For this review, take the finished solid that the model builds, in its own axes (mm). Face numbers are marked on the shaded views. A direction names the side the tool comes from. Give positions to 0.01 mm unless a question says otherwise; leave off trailing zeros. Loops run counter-clockwise (first coordinate to the right, second up) from the corner with the lowest first, then second, coordinate; pieces in that order, holes last. Notation, with made-up numbers: (80, -37.75) -> (108, -37.75) arc R15 ccw to (108, -19.75) -> close; hole circle Ø10 at (72, 19.25). An arc over 180 degrees is marked (long way). Answer as CSV lines item,"result". Start each with the question number.
Item 1: Add section D-D on y = 12.5. State the section outline as (x, z) points, plus the area to 3 significant figures.
Item 2: Machinability: for the marked faces 4, 5 and 6, which of the approach directions +Z, -Z, +X, -X, +Y, -Y give a long, thin tool a straight path to every point of the face, cutting with its end or side? Answer none if there is none.
Item 3: Clearance check with flat-ended pins moving along their axes: P1, Ø2, axis at x = 16.5, z = 13, coming from the +Y side; P2, Ø5.5, axis at x = -4, z = 16, coming from the -Y side; P3, Ø6.5, axis at y = 18.5, z = 13.5, coming from the +X side. State where each tip first meets the part, or that it passes through.
Item 4: Add section A-A on x = 0. State the section outline as (y, z) points.
Item 5: Add section B-B on y = 0. State the section outline as (x, z) points.
Item 6: Add section C-C on z = 17. State the section outline as (x, y) points.
Item 7: The part is to be moulded in two halves that separate along Y. For the marked faces 1, 2 and 3, say which applies: +Y half, -Y half, draft (parallel to the pull), parting line (faces both ways), or undercut.
Item 8: For L1, parallel to X at y = 0, z = 16.3; L2, parallel to Y at x = 16, z = 13.75; L3, parallel to Y at x = -21, z = 15, list the stretches that pass through material, from the lowest coordinate up. Write a range as from..to.
```python
from build123d import *

# Parameters (mm, degrees)
SKETCH005_R             = 30
PAD002_DEPTH            = 13
SKETCH006_R             = 29
POCKET001_DEPTH         = 3.5
SKETCH007_R             = 27.5
PAD003_DEPTH            = 3.5
SKETCH010_W             = 44
SKETCH010_H             = 22
POCKET003_DEPTH         = 7
SKETCH018_W             = 32
SKETCH018_H             = 40
POCKET011_DEPTH         = 13
SKETCH020_W             = 5
SKETCH020_H             = 3
POCKET012_DEPTH         = 8
SKETCH023_R             = 2.25
POCKET015_DEPTH         = 20
BODY002_PLACEMENT_ANGLE = 90


with BuildPart() as part:
    # Sketch005 → Pad002 (new body)
    with BuildSketch(Plane.XY):
        Circle(SKETCH005_R)
    extrude(amount=PAD002_DEPTH)

    # Sketch006 (on Face3 of Pad002) → Pocket001 (cut)
    with BuildSketch(Plane.XY.offset(13)):
        Circle(SKETCH006_R)
    extrude(amount=-POCKET001_DEPTH, mode=Mode.SUBTRACT)

    # Sketch007 (on Face5 of Pocket001) → Pad003 (join)
    with BuildSketch(Plane.XY.offset(9.5)):
        Circle(SKETCH007_R)
    extrude(amount=PAD003_DEPTH)

    # Sketch010 (on Face7 of Pad003) → Pocket003 (cut)
    with BuildSketch(Plane.XY.offset(13)):
        Rectangle(SKETCH010_W, SKETCH010_H)
    extrude(amount=-POCKET003_DEPTH, mode=Mode.SUBTRACT)

    # Sketch018 (on Face7 of Pocket003) → Pocket011 (cut)
    with BuildSketch(Plane.XY.offset(13)):
        Rectangle(SKETCH018_W, SKETCH018_H)
    extrude(amount=-POCKET011_DEPTH, mode=Mode.SUBTRACT)

    # Sketch020 (on Face5 of Pocket011) → Pocket012 (cut)
    with BuildSketch(Plane(origin=(0, -20, 0), x_dir=(-1, 0, 0), z_dir=(0, 1, 0))):
        with Locations((0, 11.5)):
            Rectangle(SKETCH020_W, SKETCH020_H)
    extrude(amount=-POCKET012_DEPTH, mode=Mode.SUBTRACT)

    # Sketch023 (on Face9 of Pocket012) → Pocket015 (cut)
    with BuildSketch(Plane.XY.offset(13)):
        with Locations((-19.108778, -14.520833)):
            Circle(SKETCH023_R)
        with Locations((0, 24)):
            Circle(SKETCH023_R)
        with Locations((19.108778, -14.520833)):
            Circle(SKETCH023_R)
    extrude(amount=-POCKET015_DEPTH, mode=Mode.SUBTRACT)


with BuildPart() as part_1:
    # Body002 placement: moved
    add(part.part.moved(Location((0, 0, 5))).rotate(Axis((0, 0, 5), (0, 0, 1)), BODY002_PLACEMENT_ANGLE))


solid = part_1.part
```
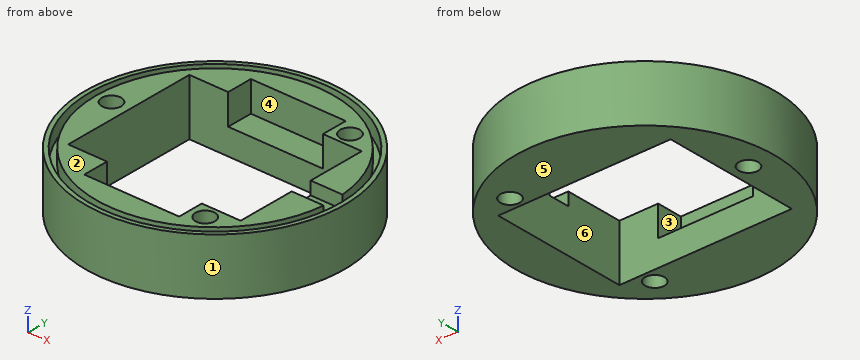
Computed values:
1,outline,"(-27.27, 5) -> (-20, 5) -> (-20, 18) -> (-24.49, 18) -> (-24.49, 14.5) -> (-26.17, 14.5) -> (-26.17, 18) -> (-27.27, 18) -> close; (20, 5) -> (27.27, 5) -> (27.27, 18) -> (26.17, 18) -> (26.17, 14.5) -> (24.49, 14.5) -> (24.49, 18) -> (20, 18) -> close"
1,area,"177 mm²"
2,face 4,"+Z"
2,face 5,"-Z, +X, -X, +Y, -Y"
2,face 6,"+Z, -Z"
3,P1,"y = 25.69"
3,P2,"y = -29.97"
3,P3,"x = 25.83"
4,outline,"(-30, 5) -> (-16, 5) -> (-16, 11) -> (-22, 11) -> (-22, 18) -> (-27.5, 18) -> (-27.5, 14.5) -> (-29, 14.5) -> (-29, 18) -> (-30, 18) -> close; (16, 5) -> (30, 5) -> (30, 18) -> (29, 18) -> (29, 14.5) -> (27.5, 14.5) -> (27.5, 18) -> (22, 18) -> (22, 11) -> (16, 11) -> close"
5,outline,"(-30, 5) -> (-26.25, 5) -> (-26.25, 18) -> (-27.5, 18) -> (-27.5, 14.5) -> (-29, 14.5) -> (-29, 18) -> (-30, 18) -> close; (-21.75, 5) -> (-20, 5) -> (-20, 18) -> (-21.75, 18) -> close; (20, 5) -> (30, 5) -> (30, 18) -> (29, 18) -> (29, 14.5) -> (27.5, 14.5) -> (27.5, 15) -> (20, 15) -> close"
6,outline,"circle Ø60 at (0, 0); (-20, -16) -> (-20, 16) -> (-11, 16) -> (-11, 22) -> (11, 22) -> (11, 16) -> (20, 16) -> (20, 2.5) -> (27.39, 2.5) arc R27.5 ccw (long way) to (27.39, -2.5) -> (20, -2.5) -> (20, -16) -> (11, -16) -> (11, -22) -> (-11, -22) -> (-11, -16) -> close; hole circle Ø58 at (0, 0); hole circle Ø4.5 at (-24, 0); hole circle Ø4.5 at (14.52, -19.11); hole circle Ø4.5 at (14.52, 19.11)"
7,face 1,"parting line"
7,face 2,"draft"
7,face 3,"undercut"
8,L1,"-30..-29, -27.5..-26.25, -21.75..-20, 29..30"
8,L2,"-25.38..-20.8, -17.41..-16, 16..17.41, 20.8..25.38"
8,L3,"-21.42..-20, -17.76..17.76, 20..21.42"
